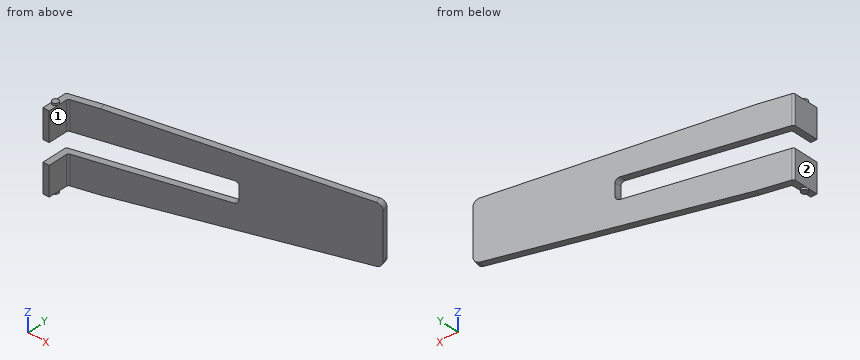
from build123d import *

# Parameters (mm, degrees)
BOSS_EXTRUDE1_DEPTH      = 3.8
CHAMFER1_SIZE            = 0.5
CHAMFER1_SIZE2           = 11.451882774
SKETCH3_R                = 0.15
BOSS_EXTRUDE2_DEPTH      = 0.1
BOSS_EXTRUDE2_DEPTH_BACK = 3.9
SKETCH4_W                = 7
SKETCH4_H                = 1
CUT_EXTRUDE2_DEPTH       = 10
FILLET1_R                = 0.1
FILLET2_R                = 0.3
FILLET3_R                = 0.2


with BuildPart() as part:
    # Sketch1 → Boss-Extrude1 (new body)
    with BuildSketch(Plane.XY):
        Polygon((0, 0), (0, 1.230198096), (12.557035742, 4.594845683), (12.634681455, 4.305067935), (0.3, 1), (0.3, 0), align=None)
    extrude(amount=BOSS_EXTRUDE1_DEPTH)

    # Chamfer1
    chamfer1_edges = [part.edges().sort_by_distance(p)[0] for p in [
        (12.595858599, 4.449956809, 3.8),
        (12.595858599, 4.449956809, 0),
    ]]
    chamfer1_side = [part.faces().sort_by_distance(p)[0] for p in [
        (12.595858599, 4.449956809, 1.9),
    ]]
    chamfer(chamfer1_edges, length=CHAMFER1_SIZE, length2=CHAMFER1_SIZE2, reference=chamfer1_side[0])

    # Sketch3 → Boss-Extrude2 (add, two sides)
    with BuildSketch(Plane.XY.offset(3.8)) as boss_extrude2_sk:
        with Locations((0.15, 0.5)):
            Circle(SKETCH3_R)
    extrude(amount=BOSS_EXTRUDE2_DEPTH)
    extrude(boss_extrude2_sk.sketch, amount=-BOSS_EXTRUDE2_DEPTH_BACK)

    # Sketch4 → Cut-Extrude2 (cut)
    with BuildSketch(Plane.XZ):
        with Locations((3.5, 1.9)):
            Rectangle(SKETCH4_W, SKETCH4_H)
    extrude(amount=-CUT_EXTRUDE2_DEPTH, mode=Mode.SUBTRACT)

    # Fillet1
    fillet1_edges = [part.edges().sort_by_distance(p)[0] for p in [
        (0, 1.230198096, 3.1),
        (0.3, 1, 3.1),
        (0, 1.230198096, 0.7),
        (0.3, 1, 0.7),
    ]]
    fillet(fillet1_edges, radius=FILLET1_R)

    # Fillet2
    fillet2_edges = [part.edges().sort_by_distance(p)[0] for p in [
        (12.595858599, 4.449956809, 0.5),
        (12.595858599, 4.449956809, 3.3),
    ]]
    fillet(fillet2_edges, radius=FILLET2_R)

    # Fillet3
    fillet3_edges = [part.edges().sort_by_distance(p)[0] for p in [
        (7, 2.950551016, 2.4),
        (7, 2.950551016, 1.4),
    ]]
    fillet(fillet3_edges, radius=FILLET3_R)


solid = part.part
Geometry check sheet. Reference: the model listing, model coordinates, mm. Face numbers are marked on the shaded views. A direction names the side the tool comes from. Give positions to 0.01 mm unless a question says otherwise; leave off trailing zeros. Loops run counter-clockwise (first coordinate to the right, second up) from the corner with the lowest first, then second, coordinate; pieces in that order, holes last.
(1) Thickness scan on L1, parallel to Z at x = 5, y = 2.3; L2, parallel to Y at x = 5.75, z = 3.15; L3, parallel to Y at x = 5.5, z = 3.2. Record the ranges inside material, lowest first.
From the geometry:
L1: z = 0.16 to 1.4, 2.4 to 3.64
L2: y = 2.46 to 2.77
L3: y = 2.39 to 2.7
(2) Depth check by flat-ended pin: pin 1 Ø0.5 at (y, z) = (0.5, 0.5) entering from +X; pin 2 Ø2.5 at (x, y) = (4.5, 2) entering from -Z; pin 3 Ø1.5 at (x, y) = (3.5, 1.5) entering from +Z. Enter the tip coordinate at first touch or a pass-through.
From the geometry:
pin 1: stops at x = 0.3
pin 2: stops at z = 0.08
pin 3: stops at z = 3.75
(3) Section check C-C on z = 1.75. Record the cut outline in (x, y).
From the geometry:
outline: (7, 2.8) - (12.63, 4.31) - (12.56, 4.59) - (7, 3.11) - close
(4) Set-up check for the marked faces 1 and 2: record each of +Z, -Z, +X, -X, +Y, -Y from which the full face is reachable in a straight line by a thin tool's end or side.
From the geometry:
face 1: +Z, -Z, +X, -Y
face 2: +Z, -Z, -X, +Y, -Y
(5) Section check A-A on x = 1.75. Record the cut outline in (y, z).
From the geometry:
outline: (1.39, 0.01) - (1.7, 0.01) - (1.7, 1.4) - (1.39, 1.4) - close; (1.39, 2.4) - (1.7, 2.4) - (1.7, 3.79) - (1.39, 3.79) - close
(6) Section check D-D on y = 3.85. Record the cut outline in (x, z), then the cut area to 3 significant figures.
From the geometry:
outline: (9.78, 0.37) - (10.94, 0.42) - (10.94, 3.38) - (9.78, 3.43) - close
area: 3.48 mm2
(7) Section check B-B on x = 4.5. Record the cut outline in (y, z).
From the geometry:
outline: (2.13, 0.13) - (2.44, 0.14) - (2.44, 1.4) - (2.13, 1.4) - close; (2.13, 2.4) - (2.44, 2.4) - (2.44, 3.66) - (2.13, 3.67) - close
